Read the model definition and answer for the solid it produces. Units are mm, in the model's axes. Face numbers are marked on the shaded views. A direction names the side the tool comes from. Give positions to 0.01 mm unless a question says otherwise; leave off trailing zeros. Order: outer loops, then holes, each group sorted by start corner. A loop starts at its lowest first (then second) coordinate and runs counter-clockwise, first axis right, second up. Notation, with made-up numbers: (60.5, -8.75) - (98.5, -8.75) arc R36 ccw to (98.5, 29.25) - close; hole circle Ø8 at (18.25, 25.5). An arc over 180 degrees is marked (long way). Use a Markdown table: item, result. Add a question column.
1. A cutting plane is placed at A-A on y = -19. Determine the outline of the cut face in (x, z).
2. A cutting plane is placed at C-C on x = -51.5. Determine the outline of the cut face in (y, z), and give its area (3 significant figures).
3. Which of the six approach directions +Z, -Z, +X, -X, +Y, -Y give full straight-line access (tool end or side, diameter ignored) to the marked faces 4 and 5?
4. Consider L1, parallel to X at y = -27.7, z = 23; L2, parallel to Z at x = -51.6, y = 19; L3, parallel to Y at x = -51.25, z = 24.75. Determine where each line is inside the solid, lowest interval first.
5. For a pull along Y with two mould halves and no side action, classify the marked faces 1, 2 and 3 as released by +Y, released by -Y, zero draft, split by the parting line, or undercut.
6. A cutting plane is placed at D-D on z = 25.75. Determine the outline of the cut face in (x, y), and give its area (3 significant figures).
7. A cutting plane is placed at B-B on z = 22.5. Determine the outline of the cut face in (x, y).
8. A flat-ended cylindrical pin translates along its axis: P1, Ø2.5, axis at x = -51.5, z = 23, coming from the +Y side. Find the tip coordinate at first contact, or state that the pin passes through.
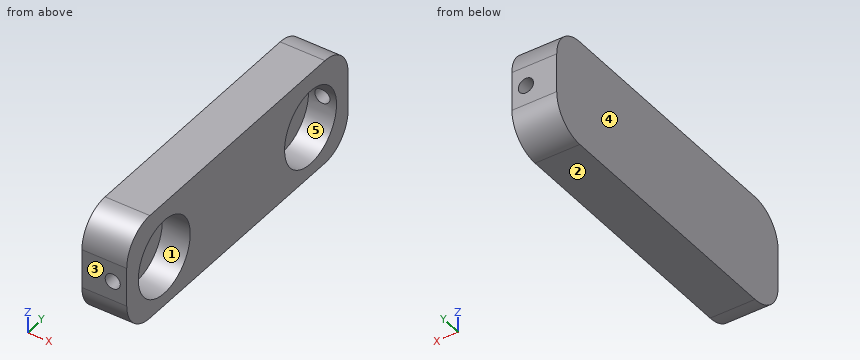
```python
from build123d import *

# Parameters (mm, degrees)
BOX008_W          = 10
BOX008_H          = 64
BOX008_DEPTH      = 42
BOX006_W          = 5
BOX006_H          = 57.5
BOX006_DEPTH      = 19
FILLET008_R       = 6
CYLINDER027_R     = 1.35
CYLINDER027_DEPTH = 10
CYLINDER025_R     = 1.35
CYLINDER025_DEPTH = 10
CYLINDER028_R     = 6.75
CYLINDER028_DEPTH = 50
CYLINDER026_R     = 6.75
CYLINDER026_DEPTH = 50
BOX007_W          = 5
BOX007_H          = 57.5
BOX007_DEPTH      = 19
FILLET009_R       = 6


with BuildPart() as cube008:
    # Box008 → Box008 (new body)
    with BuildSketch(Plane(origin=(-32, -32, 0), x_dir=(1, 0, 0), z_dir=(0, 0, 1))):
        with Locations((5, 32)):
            Rectangle(BOX008_W, BOX008_H)
    extrude(amount=BOX008_DEPTH)


with BuildPart() as cut024:
    # Box006 → Box006 (new body)
    with BuildSketch(Plane(origin=(0, -28.75, 13.5), x_dir=(1, 0, 0), z_dir=(0, 0, 1))):
        with Locations((2.5, 28.75)):
            Rectangle(BOX006_W, BOX006_H)
    extrude(amount=BOX006_DEPTH)

    # Fillet008
    fillet008_edges = [cut024.edges().sort_by_distance(p)[0] for p in [
        (2.5, -28.75, 13.5),
        (2.5, -28.75, 32.5),
        (2.5, 28.75, 13.5),
        (2.5, 28.75, 32.5),
    ]]
    fillet(fillet008_edges, radius=FILLET008_R)


with BuildPart() as cut024_1:
    # Fillet008 placement: moved
    add(cut024.part.moved(Location((-24, 0, 0))))

    # Cut024: cut Cube008
    add(cube008.part, mode=Mode.SUBTRACT)


with BuildPart() as cut024_2:
    # Cut024 placement: moved
    add(cut024_1.part.moved(Location((19, 0, 0))))


with BuildPart() as cylinder019:
    # Cylinder027 → Cylinder027 (new body)
    with BuildSketch(Plane(origin=(2.5, -22, 23), x_dir=(1, 0, 0), z_dir=(0, -1, 0))):
        Circle(CYLINDER027_R)
    extrude(amount=CYLINDER027_DEPTH)


with BuildPart() as cylinder018:
    # Cylinder025 → Cylinder025 (new body)
    with BuildSketch(Plane(origin=(2.5, 32, 23), x_dir=(1, 0, 0), z_dir=(0, -1, 0))):
        Circle(CYLINDER025_R)
    extrude(amount=CYLINDER025_DEPTH)


with BuildPart() as tubo008:
    # Cylinder028 → Cylinder028 (new body)
    with BuildSketch(Plane(origin=(-24, 19, 22.5), x_dir=(0, 0, -1), z_dir=(1, 0, 0))):
        Circle(CYLINDER028_R)
    extrude(amount=CYLINDER028_DEPTH)


with BuildPart() as tubo007:
    # Cylinder026 → Cylinder026 (new body)
    with BuildSketch(Plane(origin=(-24, -19, 22.5), x_dir=(0, 0, -1), z_dir=(1, 0, 0))):
        Circle(CYLINDER026_R)
    extrude(amount=CYLINDER026_DEPTH)


with BuildPart() as obj1:
    # Box007 → Box007 (new body)
    with BuildSketch(Plane(origin=(0, -28.75, 13.5), x_dir=(1, 0, 0), z_dir=(0, 0, 1))):
        with Locations((2.5, 28.75)):
            Rectangle(BOX007_W, BOX007_H)
    extrude(amount=BOX007_DEPTH)

    # Fillet009
    fillet009_edges = [obj1.edges().sort_by_distance(p)[0] for p in [
        (2.5, -28.75, 13.5),
        (2.5, -28.75, 32.5),
        (2.5, 28.75, 13.5),
        (2.5, 28.75, 32.5),
    ]]
    fillet(fillet009_edges, radius=FILLET009_R)

    # Cut022: cut tubo007
    add(tubo007.part, mode=Mode.SUBTRACT)

    # Cut020: cut tubo008
    add(tubo008.part, mode=Mode.SUBTRACT)

    # Cut023: cut Cylinder018
    add(cylinder018.part, mode=Mode.SUBTRACT)

    # Cut021: cut Cylinder019
    add(cylinder019.part, mode=Mode.SUBTRACT)

    # Fusion007: union Cut024
    add(cut024_2.part)


with BuildPart() as obj1_1:
    # Fusion007 placement: moved
    add(obj1.part.moved(Location((-54, 0, 0))))


solid = obj1_1.part
```
Output values:
| question | item | result |
|---|---|---|
| 1 | outline | (-57, 13.5) - (-49, 13.5) - (-49, 15.75) - (-54, 15.75) - (-54, 29.25) - (-49, 29.25) - (-49, 32.5) - (-57, 32.5) - close |
| 2 | outline | (-28.75, 19.5) arc R6 ccw to (-22.75, 13.5) - (22.75, 13.5) arc R6 ccw to (28.75, 19.5) - (28.75, 21.65) - (25.7, 21.65) arc R6.75 cw (long way) to (25.49, 24.35) - (28.75, 24.35) - (28.75, 26.5) arc R6 ccw to (22.75, 32.5) - (-22.75, 32.5) arc R6 ccw to (-28.75, 26.5) - (-28.75, 24.35) - (-25.49, 24.35) arc R6.75 cw (long way) to (-25.7, 21.65) - (-28.75, 21.65) - close |
| 2 | area | 759 mm² |
| 3 | face 4 | +Z, -Z, -X, +Y, -Y |
| 3 | face 5 | +X |
| 4 | L1 | -57 to -52.85, -50.15 to -49 |
| 4 | L2 | 13.5 to 15.75, 29.25 to 32.5 |
| 4 | L3 | -28.75 to -25.36, -12.64 to 12.64, 25.36 to 28.75 |
| 5 | face 1 | undercut |
| 5 | face 2 | zero draft |
| 5 | face 3 | released by -Y |
| 6 | outline | (-57, -28.75) - (-49, -28.75) - (-49, -24.92) - (-54, -24.92) - (-54, -13.08) - (-49, -13.08) - (-49, 13.08) - (-54, 13.08) - (-54, 24.92) - (-49, 24.92) - (-49, 28.75) - (-57, 28.75) - close |
| 6 | area | 342 mm² |
| 7 | outline | (-57, -28.75) - (-52.75, -28.75) - (-52.75, -25.75) - (-54, -25.75) - (-54, -12.25) - (-49, -12.25) - (-49, 12.25) - (-54, 12.25) - (-54, 25.75) - (-52.75, 25.75) - (-52.75, 28.75) - (-57, 28.75) - close; (-50.25, -28.75) - (-49, -28.75) - (-49, -25.75) - (-50.25, -25.75) - close; (-50.25, 25.75) - (-49, 25.75) - (-49, 28.75) - (-50.25, 28.75) - close |
| 8 | P1 | y = 12.48 |
